from build123d import *

# Parameters (mm, degrees)
SKETCH_R     = 19.35
PAD_DEPTH    = 33.5
SKETCH001_R  = 10
PAD001_DEPTH = 5
SKETCH002_R  = 3
PAD002_DEPTH = 12.5
SKETCH003_R  = 1.5
POCKET_DEPTH = 10


with BuildPart() as part:
    # Sketch → Pad (new body)
    with BuildSketch(Plane.XZ):
        Circle(SKETCH_R)
    extrude(amount=PAD_DEPTH)

    # Sketch001 (on Face3 of Pad) → Pad001 (join)
    with BuildSketch(Plane.XZ.offset(33.5)):
        Circle(SKETCH001_R)
    extrude(amount=PAD001_DEPTH)

    # Sketch002 (on Face5 of Pad001) → Pad002 (join)
    with BuildSketch(Plane.XZ.offset(38.5)):
        Circle(SKETCH002_R)
    extrude(amount=PAD002_DEPTH)

    # Sketch003 (on Face3 of Pad002) → Pocket (cut)
    with BuildSketch(Plane.XZ.offset(33.5)):
        with Locations((14, 0)):
            Circle(SKETCH003_R)
        with Locations((-12.990382, -7.499998)):
            Circle(SKETCH003_R)
        with Locations((-6.999999, -12.124356)):
            Circle(SKETCH003_R)
        with Locations((12.990379, -7.500003)):
            Circle(SKETCH003_R)
        with Locations((0, 15)):
            Circle(SKETCH003_R)
        with Locations((-6.999999, 12.124356)):
            Circle(SKETCH003_R)
    extrude(amount=-POCKET_DEPTH, mode=Mode.SUBTRACT)


solid = part.part
Model file for the job. Use its own axes, mm. A direction names the side the tool comes from. Give positions to 0.01 mm unless a question says otherwise; leave off trailing zeros. Order: outer loops, then holes, each group sorted by start corner. A loop starts at its lowest first (then second) coordinate and runs counter-clockwise, first axis right, second up. Notation, with made-up numbers: M -11.75,38 L 43.25,38 A25 ccw 43.25,56 Z; hole C -6,72.5 d4. An arc over 180 degrees is marked long. Put each result on its own line as item: value. Start each with the question number.
(1) Drill centre lines: L1, parallel to Y at x = -6, z = 16.5; L2, parallel to X at y = -18, z = -0.5; L3, parallel to Y at x = -0.5, z = 15. Where is each one in solid material? Low to high. Write a range as [from, to].
(2) Band-saw the part on A-A on z = 0. Give the cut face in (x, y).
(3) Band-saw the part on B-B on y = -28. Give the cut face in (x, z), then the cut area to 3 significant figures.
(4) Band-saw the part on D-D on y = -7.5. Give the cut face in (x, z), then the cut area to 3 significant figures.
(5) Tool access for faces 4 (the face through (-19.33, -16.52, 0.85)), 5 (the face through (-12.3, -28.57, -8.83)): list every direction of +Z, -Z, +X, -X, +Y, -Y with a clear straight run to the whole face (end or side of a thin tool).
(6) Band-saw the part on C-C on x = -7. Give the cut face in (y, z), then the cut area to 3 significant figures.
(7) Pin check, flat tips, straight feed: pin 1 Ø3.5 at (x, z) = (-6.5, -12.5) entering from -Y; pin 2 Ø0.9 at (x, z) = (-12.5, -8) entering from -Y; pin 3 Ø6 at (x, y) = (-10, -28.5) entering from -Z; pin 4 Ø1 at (x, z) = (-11, 2) entering from +Y. Stop position of each tip, or through.
(8) Pull direction Z, two halves, no side cores. Call faces 1 (the face through (-2.17, -35.97, -9.76)), 2 (the face through (0, -51, 0)), 3 (the face through (-13, -23.5, -7)): released by +Z, released by -Z, zero draft, split by the parting line, or undercut.
Results below:
1. L1: y = [-33.5, 0]
1. L2: x = [-19.34, 19.34]
1. L3: y = [-23.5, 0]
2. outline: M -19.35,-33.5 L -10,-33.5 L -10,-38.5 L -3,-38.5 L -3,-51 L 3,-51 L 3,-38.5 L 10,-38.5 L 10,-33.5 L 12.5,-33.5 L 12.5,-23.5 L 15.5,-23.5 L 15.5,-33.5 L 19.35,-33.5 L 19.35,0 L -19.35,0 Z
3. outline: C 0,0 d38.7; hole C -12.99,-7.5 d3; hole C -7,-12.12 d3; hole C -7,12.12 d3; hole C 0,15 d3; hole C 12.99,-7.5 d3; hole C 14,0 d3
3. area: 1,130 mm2
4. outline: C 0,0 d38.7
4. area: 1,180 mm2
5. face 4: +Y, -Y
5. face 5: -Y
6. outline: M -38.5,-7.14 L -33.5,-7.14 L -33.5,-10.62 L -23.5,-10.62 L -23.5,-13.62 L -33.5,-13.62 L -33.5,-18.04 L 0,-18.04 L 0,18.04 L -33.5,18.04 L -33.5,13.62 L -23.5,13.62 L -23.5,10.62 L -33.5,10.62 L -33.5,7.14 L -38.5,7.14 Z
6. area: 1,220 mm2
7. pin 1: stops at y = -33.5
7. pin 2: stops at y = -23.5
7. pin 3: stops at z = -18.04
7. pin 4: stops at y = 0
8. face 1: split by the parting line
8. face 2: zero draft
8. face 3: undercut
